For this review, take the finished solid that the model builds, in its own axes (mm). A direction names the side the tool comes from. Give positions to 0.01 mm unless a question says otherwise; leave off trailing zeros. Write each loop counter-clockwise with the first axis right and the second up, starting at its lowest first coordinate (ties: lowest second). Pieces come first, ordered by that corner, then holes. Notation, with made-up numbers: M 39.5,53 L 95.5,53 A20 ccw 95.5,78 Z; hole C -24.5,17 d8. An arc over 180 degrees is marked long. Write item = value, one per line.
Autodesk Inventor part; units mm, degrees
ref_plane "Arbeitsebene1" through (0, 0, 0) normal (1, 0, 0) x (0, 1, 0)
ref_plane "XZ Plane" through (0, 0, 0) normal (0, 1, 0) x (-1, 0, 0)
ref_plane "XY Plane" through (0, 0, 0) normal (0, 0, 1) x (1, 0, 0)
sketch "Skizze1" plane through (0, 0, 0) normal (0, 0, 1) x (1, 0, 0)
  line L0 (-34.75, -27.5) -> (34.75, -27.5)
  line L1 (34.75, -27.5) -> (34.75, 27.5)
  line L2 (34.75, 27.5) -> (-34.75, 27.5)
  line L3 (-34.75, 27.5) -> (-34.75, -27.5)
  line L4 (-34.75, -27.5) -> (34.75, 27.5) construction
  line L5 (34.75, -27.5) -> (-34.75, 27.5) construction
  point P0 (0, 0)
  dimension "d0" = 69.5
  dimension "d1" = 55
extrude "Extrusion1" add sketch "Skizze1" against normal blind 33
sketch "Skizze2" plane through (0, 0, 0) normal (0, 0, 1) x (1, 0, 0)
  line L0 (-34.75, 27.5) -> (-34.75, -27.5)
  line L1 (-34.75, -27.5) -> (34.75, -27.5)
  point P0 (0, 0)
  point P1 (-19.75, 11.5)
  dimension "d11" = 15
  dimension "d12" = 39
hole "Bohrung1" at (-19.75, 11.5, 0) direction (0, 0, -1) diameter 17.294 depth 23 tip angle 118
sketch "Skizze4" plane through (34.75, -27.5, 0) normal (1, 0, 0) x (0, 0, -1)
  line L0 (0, 0) -> (33, 0)
  line L1 (33, 55) -> (33, 0)
  point P0 (0, 27.5)
  point P1 (6, 49)
  point P2 (14, 49)
  point P3 (6, 29)
  point P4 (14, 29)
  dimension "d21" = 29
  dimension "d22" = 20
  dimension "d23" = 27
  dimension "d24" = 27
  dimension "d85" = 8
hole "Bohrung3" at (34.75, 21.5, -14) at (34.75, 1.5, -14) direction (-1, 0, 0) diameter 4.134 depth 15 tip angle 118
hole "Bohrung4" at (34.75, 21.5, -6) at (34.75, 1.5, -6) direction (-1, 0, 0) diameter 3 depth 8 tip angle 118
sketch "Skizze5" plane through (34.75, -27.5, 0) normal (1, 0, 0) x (0, 0, -1)
  line L0 (33, 55) -> (33, 0)
  line L1 (0, 0) -> (0, 55)
  line L2 (0, 42) -> (33, 42) construction
  line L3 (0, 55) -> (33, 55)
  point P0 (0, 27.5)
  point P1 (26.5, 42)
  point P2 (16.5, 42)
  dimension "d48" = 6.5
  dimension "d49" = 13
hole "Bohrung5" at (34.75, 14.5, -26.5) direction (-1, 0, 0) diameter 4 depth 50 counterbore diameter 10 counterbore depth 1.5
sketch "Skizze6" plane through (-34.75, -27.5, 0) normal (0, -1, 0) x (1, 0, 0)
  line L0 (69.5, -33) -> (0, -33)
  line L1 (69.5, 0) -> (69.5, -33)
  line L2 (69.5, -16.5) -> (0, -16.5) construction
  point P0 (34.75, 0)
  point P1 (60.5, -27)
  point P2 (60.5, -9)
  dimension "d57" = 6
  dimension "d58" = 18
  dimension "d59" = 9
  dimension "d60" = 9
hole "Bohrung6" at (25.75, -27.5, -27) at (25.75, -27.5, -9) direction (0, 1, 0) diameter 3.2 depth 8 tip angle 118
sketch "Skizze7" plane through (-34.75, -27.5, 0) normal (0, -1, 0) x (1, 0, 0)
  circle A0 centre (60.5, -27) radius 1.6
  line L0 (69.5, 0) -> (69.5, -33)
  point P0 (34.75, 0)
  point P1 (60.5, -16.5)
  point P2 (69.5, -16.5)
hole "Bohrung7" at (25.75, -27.5, -16.5) direction (0, 1, 0) diameter 4.134 depth 17 tip angle 118
ref_plane "Arbeitsebene1" through (0, 0, 0) normal (1, 0, 0) x (0, 1, 0)
mirror "Spiegeln1" about plane through (0, 0, 0) normal (1, 0, 0) of "Bohrung6"
sketch "Skizze8" plane through (-34.75, -27.5, 0) normal (0, -1, 0) x (1, 0, 0)
  line L0 (69.5, 0) -> (69.5, -33)
  line L1 (0, 0) -> (0, -33)
  line L2 (69.5, 0) -> (69.5, -33)
  line L3 (0, 0) -> (69.5, 0)
  point P0 (34.75, 0)
  point P1 (29, -16.5)
  point P2 (69.5, -16.5)
  point P3 (69.5, -16.5)
  dimension "d76" = 29
  dimension "d77" = 16.5
hole "Bohrung8" at (-5.75, -27.5, -16.5) direction (0, 1, 0) diameter 4.134 depth 17 tip angle 118
chamfer "Fasen1" distance 0.5 angle 45 11 edges at (34.75, 0, 0) (0, 27.5, 0) (-34.75, 0, 0) (0, -27.5, 0) (34.75, -27.5, -16.5) (34.75, 0, -33) (34.75, 27.5, -16.5) (-34.75, 27.5, -16.5) (0, 27.5, -33) (0, -27.5, -33) (-34.75, -27.5, -16.5)
chamfer "Fasen2" distance 0.5 angle 45 1 edges at (-34.75, 0, -33)
properties part number "Steuerblock" material "Stahl, Legierung"
1. For line 1 along Y through (x, z) = (26, -14); line 2 along Z through (x, y) = (28.5, 1.5); line 3 along X through (y, z) = (-22.5, -27), list the stretches that pass through material, from the lowest coordinate up. Write a range as from..to.
Responses:
line_1 = -27.5..-0.57, 3.57..19.43, 23.57..27.5
line_2 = -33..-16.07, -11.93..-7.5, -4.5..0
line_3 = -34.75..-27.35, -24.15..24.15, 27.35..34.75
2. We need section B-B, the plane x = 22. Write out the cut boundary in (y, z), then the cut area to 3 significant figures.
Responses:
outline = M -27.5,-32.5 L -27,-33 L 27,-33 L 27.5,-32.5 L 27.5,-0.5 L 27,0 L -27,0 L -27.5,-0.5 Z; hole C 1.5,-14 d4.13; hole C 14.5,-26.5 d4; hole C 21.5,-14 d4.13
area = 1,780 mm2
3. We need section A-A, the plane z = -3. Write out the cut boundary in (x, y).
Responses:
outline = M -34.75,-27 L -34.25,-27.5 L 34.25,-27.5 L 34.75,-27 L 34.75,27 L 34.25,27.5 L -34.25,27.5 L -34.75,27 Z; hole C -19.75,11.5 d17.29
4. Insertion check: P1, Ø9, axis at y = 14.5, z = -26.5, coming from the +X side; P2, Ø5, axis at x = -5.75, z = -16.5, coming from the -Y side; P3, Ø14, axis at x = -19.75, y = 11.5, coming from the +Z side; P4, Ø1.2, axis at y = 14, z = -27, coming from the +X side. Each pin has a flat end and moves straight along its axis. Give the tip position at first contact, or say it passes through.
Responses:
P1 = 33.25
P2 = -27.5
P3 = -23.99
P4 = -15.25
5. The part is to be moulded in two halves that separate along X. For faces 1 (the face through (-5.7, -9.5, -16.1)), 2 (the face through (30.7, 2.4, -4.8)), 3 (the face through (-26, -18.7, -27.1)), 4 (the face through (-15.25, 14, -27)), say which applies: +X half, -X half, draft (parallel to the pull), parting line (faces both ways), or undercut.
Responses:
face_1 = undercut
face_2 = draft
face_3 = undercut
face_4 = +X half
6. Machinability: for faces 5 (the face through (-7.5, -18.9, -17.6)), 6 (the face through (0, 27.5, -16)), 7 (the face through (8.66, 13.899, -28.408)), which of the approach directions +Z, -Z, +X, -X, +Y, -Y give a long, thin tool a straight path to every point of the face, cutting with its end or side? Answer none if there is none.
Responses:
face_5 = -Y
face_6 = +Z, -Z, +X, -X, +Y
face_7 = +X
